Geometry: final body of the model. Coordinates: model frame, mm. Give positions to 0.01 mm unless a question says otherwise; leave off trailing zeros. Write each loop counter-clockwise with the first axis right and the second up, starting at its lowest first coordinate (ties: lowest second). Pieces come first, ordered by that corner, then holes.
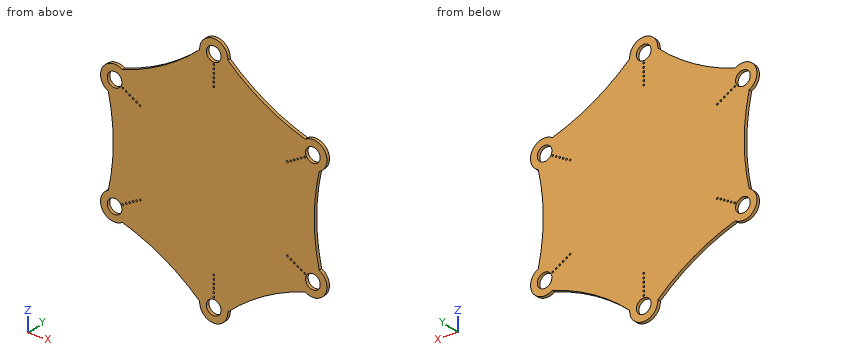
```python
from build123d import *

# Parameters (mm, degrees)
ESBO_O1_R                = 3.65
RESSALTO_EXTRUS_O1_DEPTH = 1.6
ESBO_O3_R                = 0.0001
RESSALTO_EXTRUS_O3_DEPTH = 0.001
ESBO_O5_R                = 0.45
CORTE_EXTRUS_O2_DEPTH    = 1.6


with BuildPart() as part:
    # Esboço1 → Ressalto-extrusão1 (new body)
    with BuildSketch(Plane(origin=(0, 0, 0), x_dir=(1, 0, 0), z_dir=(0, 1, 0))):
        with BuildLine():
            ThreePointArc((-52.484604611, -22.234349076), (-50.025216279, 0), (-52.484604611, 22.234349076))
            ThreePointArc((-52.484604611, 22.234349076), (-55.425625842, 32), (-45.497813442, 34.335826363))
            ThreePointArc((-45.497813442, 34.335826363), (-25.01260814, 43.323108128), (-6.98679117, 56.570175439))
            ThreePointArc((-6.98679117, 56.570175439), (0, 64), (6.98679117, 56.570175439))
            ThreePointArc((6.98679117, 56.570175439), (25.01260814, 43.323108128), (45.497813442, 34.335826363))
            ThreePointArc((45.497813442, 34.335826363), (55.425625842, 32), (52.484604611, 22.234349076))
            ThreePointArc((52.484604611, 22.234349076), (50.025216279, 0), (52.484604611, -22.234349076))
            ThreePointArc((52.484604611, -22.234349076), (55.425625842, -32), (45.497813442, -34.335826363))
            ThreePointArc((45.497813442, -34.335826363), (25.01260814, -43.323108128), (6.98679117, -56.570175439))
            ThreePointArc((6.98679117, -56.570175439), (0, -64), (-6.98679117, -56.570175439))
            ThreePointArc((-6.98679117, -56.570175439), (-25.01260814, -43.323108128), (-45.497813442, -34.335826363))
            ThreePointArc((-45.497813442, -34.335826363), (-55.425625842, -32), (-52.484604611, -22.234349076))
        make_face()
        with Locations(Location((-49.363448016, 28.5, 0), (0, 0, 270))):
            Circle(ESBO_O1_R, mode=Mode.SUBTRACT)
        with Locations(Location((-49.363448016, -28.5, 0), (0, 0, 270))):
            Circle(ESBO_O1_R, mode=Mode.SUBTRACT)
        with Locations(Location((0, -57, 0), (0, 0, 270))):
            Circle(ESBO_O1_R, mode=Mode.SUBTRACT)
        with Locations(Location((49.363448016, -28.5, 0), (0, 0, 270))):
            Circle(ESBO_O1_R, mode=Mode.SUBTRACT)
        with Locations(Location((49.363448016, 28.5, 0), (0, 0, 270))):
            Circle(ESBO_O1_R, mode=Mode.SUBTRACT)
        with Locations(Location((0, 57, 0), (0, 0, 270))):
            Circle(ESBO_O1_R, mode=Mode.SUBTRACT)
    extrude(amount=RESSALTO_EXTRUS_O1_DEPTH)

    # Esboço3 → Ressalto-extrusão3 (add)
    with BuildSketch(Plane(origin=(0, 1.6, 0), x_dir=(1, 0, 0), z_dir=(0, 1, 0))):
        with Locations(Location((0, 0, 0), (0, 0, 270))):
            Circle(ESBO_O3_R)
    extrude(amount=RESSALTO_EXTRUS_O3_DEPTH)

    # Esboço5 → Corte-extrusão2 (cut)
    with BuildSketch(Plane(origin=(0, 1.6, 0), x_dir=(1, 0, 0), z_dir=(0, 1, 0))):
        with Locations(Location((0, -52.32, 0), (0, 0, 270))):
            Circle(ESBO_O5_R)
        with Locations(Location((-45.310449126, -26.16, 0), (0, 0, 270))):
            Circle(ESBO_O5_R)
        with Locations(Location((-45.310449126, 26.16, 0), (0, 0, 270))):
            Circle(ESBO_O5_R)
        with Locations(Location((0, 52.32, 0), (0, 0, 270))):
            Circle(ESBO_O5_R)
        with Locations(Location((45.310449126, 26.16, 0), (0, 0, 270))):
            Circle(ESBO_O5_R)
        with Locations(Location((45.310449126, -26.16, 0), (0, 0, 270))):
            Circle(ESBO_O5_R)
        with Locations(Location((0, -50.32, 0), (0, 0, 270))):
            Circle(ESBO_O5_R)
        with Locations(Location((0, -48.32, 0), (0, 0, 270))):
            Circle(ESBO_O5_R)
        with Locations(Location((0, -46.32, 0), (0, 0, 270))):
            Circle(ESBO_O5_R)
        with Locations(Location((0, -44.32, 0), (0, 0, 270))):
            Circle(ESBO_O5_R)
        with Locations(Location((0, -42.32, 0), (0, 0, 270))):
            Circle(ESBO_O5_R)
        with Locations(Location((-36.650195088, -21.16, 0), (0, 0, 270))):
            Circle(ESBO_O5_R)
        with Locations(Location((-38.382245896, -22.16, 0), (0, 0, 270))):
            Circle(ESBO_O5_R)
        with Locations(Location((-40.114296703, -23.16, 0), (0, 0, 270))):
            Circle(ESBO_O5_R)
        with Locations(Location((-41.846347511, -24.16, 0), (0, 0, 270))):
            Circle(ESBO_O5_R)
        with Locations(Location((-43.578398318, -25.16, 0), (0, 0, 270))):
            Circle(ESBO_O5_R)
        with Locations(Location((-36.650195088, 21.16, 0), (0, 0, 270))):
            Circle(ESBO_O5_R)
        with Locations(Location((-38.382245896, 22.16, 0), (0, 0, 270))):
            Circle(ESBO_O5_R)
        with Locations(Location((-40.114296703, 23.16, 0), (0, 0, 270))):
            Circle(ESBO_O5_R)
        with Locations(Location((-41.846347511, 24.16, 0), (0, 0, 270))):
            Circle(ESBO_O5_R)
        with Locations(Location((-43.578398318, 25.16, 0), (0, 0, 270))):
            Circle(ESBO_O5_R)
        with Locations(Location((0, 42.32, 0), (0, 0, 270))):
            Circle(ESBO_O5_R)
        with Locations(Location((0, 44.32, 0), (0, 0, 270))):
            Circle(ESBO_O5_R)
        with Locations(Location((0, 46.32, 0), (0, 0, 270))):
            Circle(ESBO_O5_R)
        with Locations(Location((0, 48.32, 0), (0, 0, 270))):
            Circle(ESBO_O5_R)
        with Locations(Location((0, 50.32, 0), (0, 0, 270))):
            Circle(ESBO_O5_R)
        with Locations(Location((36.650195088, 21.16, 0), (0, 0, 270))):
            Circle(ESBO_O5_R)
        with Locations(Location((38.382245896, 22.16, 0), (0, 0, 270))):
            Circle(ESBO_O5_R)
        with Locations(Location((40.114296703, 23.16, 0), (0, 0, 270))):
            Circle(ESBO_O5_R)
        with Locations(Location((41.846347511, 24.16, 0), (0, 0, 270))):
            Circle(ESBO_O5_R)
        with Locations(Location((43.578398318, 25.16, 0), (0, 0, 270))):
            Circle(ESBO_O5_R)
        with Locations(Location((36.650195088, -21.16, 0), (0, 0, 270))):
            Circle(ESBO_O5_R)
        with Locations(Location((38.382245896, -22.16, 0), (0, 0, 270))):
            Circle(ESBO_O5_R)
        with Locations(Location((40.114296703, -23.16, 0), (0, 0, 270))):
            Circle(ESBO_O5_R)
        with Locations(Location((41.846347511, -24.16, 0), (0, 0, 270))):
            Circle(ESBO_O5_R)
        with Locations(Location((43.578398318, -25.16, 0), (0, 0, 270))):
            Circle(ESBO_O5_R)
    extrude(amount=-CORTE_EXTRUS_O2_DEPTH, mode=Mode.SUBTRACT)


solid = part.part
```
Item 1: Section B-B, the plane x = 2. Return the cut outline in (y, z), plus the area to 3 significant figures.
Found:
outline: (0, -63.71) - (1.6, -63.71) - (1.6, -60.05) - (0, -60.05) - close; (0, -53.95) - (1.6, -53.95) - (1.6, 53.95) - (0, 53.95) - close; (0, 60.05) - (1.6, 60.05) - (1.6, 63.71) - (0, 63.71) - close
area: 184 mm2
Item 2: Section D-D, the plane z = -11. Return the cut outline in (x, y), plus the area to 3 significant figures.
Found:
outline: (-50.62, 0) - (50.62, 0) - (50.62, 1.6) - (-50.62, 1.6) - close
area: 162 mm2
Item 3: Section C-C, the plane y = 1.1. State how many separate pieces and enclosed holes the cut face has, plus the area to 3 significant figures.
Found:
separate pieces: 1
enclosed holes: 42
area: 9,160 mm2
Item 4: Line query: L1, parallel to X at y = 0.6, z = -24.5; L2, parallel to Z at x = 47, y = 0.6; L3, parallel to Z at x = -48, y = 1.35. Output: solid intervals per line, ascending.
Found:
L1: x = -55.11 to -42.14, -41.55 to 41.55, 42.14 to 55.11
L2: z = -35.09 to -31.28, -25.72 to 25.72, 31.28 to 35.09
L3: z = -35.37 to -31.89, -25.11 to 25.11, 31.89 to 35.37
Item 5: Section A-A, the plane z = 28.5. Return the cut outline in (x, y), plus the area to 3 significant figures.
Found:
outline: (-56.36, 0) - (-53.01, 0) - (-53.01, 1.6) - (-56.36, 1.6) - close; (-45.71, 0) - (45.71, 0) - (45.71, 1.6) - (-45.71, 1.6) - close; (53.01, 0) - (56.36, 0) - (56.36, 1.6) - (53.01, 1.6) - close
area: 157 mm2
